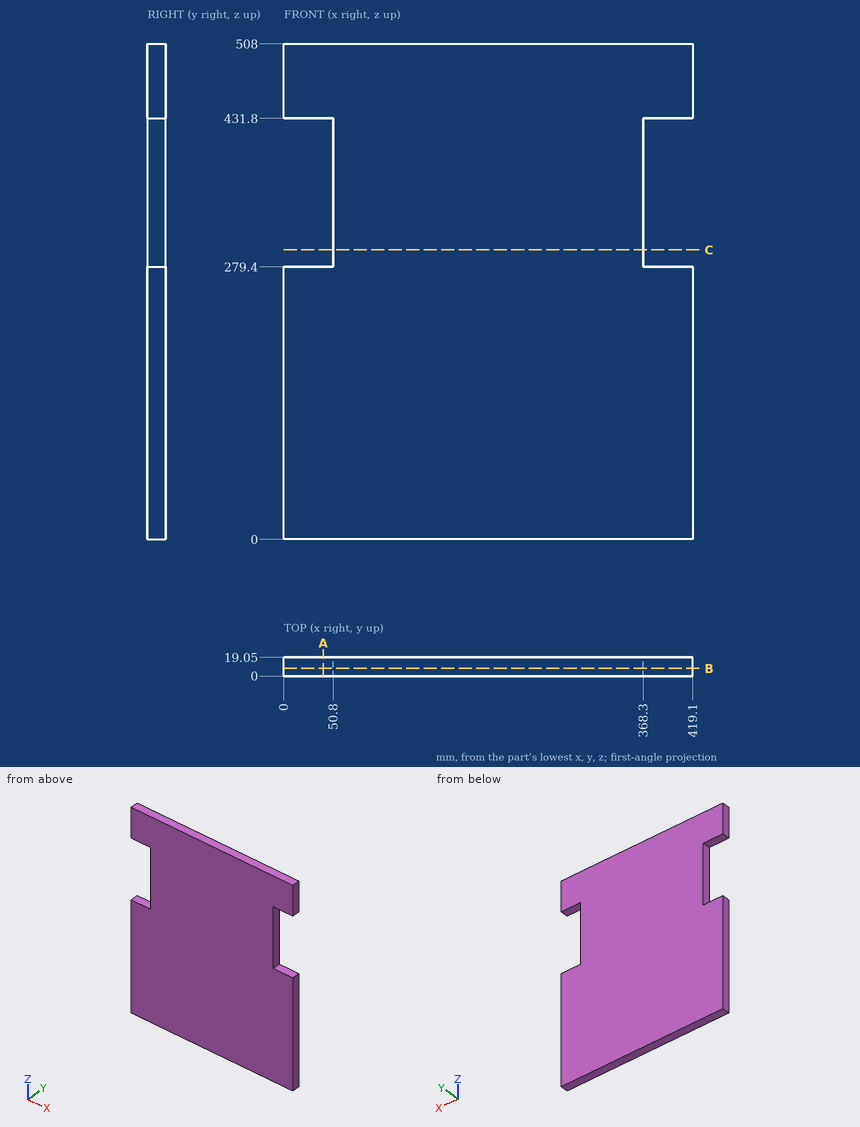
Study the drawing (mm; zero at the part's minimum x, y, z) and answer. Give positions to 0.01 mm unless a question says otherwise; leave off trailing zeros. Loops run counter-clockwise (first coordinate to the right, second up) from the corner with the lowest first, then second, coordinate; pieces in that order, holes last. Notation, with made-up numbers: (61.5, 82.5) - (118.5, 82.5) arc R17 cw to (118.5, 88.5) - close; hole circle Ø6 at (-40, 26.5). An arc over 180 degrees is marked (long way). Return JSON: item names as keys, results as strings. Group by question number.
1. Given pin 1 Ø9.5 at (y, z) = (11.5, 377.5) entering from +X, flat-ended and moving along its own axis, determine where the tip first touches the part or whether it passes through.
2. Find section A-A (x = 40.5). Write down the section's boundary in (y, z).
3. Find section C-C (z = 297). Write down the section's boundary in (x, y), then the cut area to 3 significant figures.
4. Find section B-B (y = 7.75). Write down the section's boundary in (x, z).
5. Straight lines are drawn through the part: line 1 (Z direction, x = 37, y = 2.75); line 2 (X direction, y = 7, z = 357.5). For each, find the intervals that lie inside material, in ascending order. Write a range as [from, to].
Verdict:
{
 "1": {"pin 1": "stops at x = 368.3"},
 "2": {"outline": "(0, 0) - (19.05, 0) - (19.05, 279.4) - (0, 279.4) - close; (0, 431.8) - (19.05, 431.8) - (19.05, 508) - (0, 508) - close"},
 "3": {"outline": "(50.8, 0) - (368.3, 0) - (368.3, 19.05) - (50.8, 19.05) - close", "area": "6,050 mm^2"},
 "4": {"outline": "(0, 0) - (419.1, 0) - (419.1, 279.4) - (368.3, 279.4) - (368.3, 431.8) - (419.1, 431.8) - (419.1, 508) - (0, 508) - (0, 431.8) - (50.8, 431.8) - (50.8, 279.4) - (0, 279.4) - close"},
 "5": {"line 1": "z = [0, 279.4], [431.8, 508]", "line 2": "x = [50.8, 368.3]"}
}
